Autodesk Inventor part; units mm, degrees
ref_plane "YZ Plane" through (0, 0, 0) normal (1, 0, 0) x (0, 1, 0)
ref_plane "XZ Plane" through (0, 0, 0) normal (0, 1, 0) x (-1, 0, 0)
ref_plane "XY Plane" through (0, 0, 0) normal (0, 0, 1) x (1, 0, 0)
sketch "Sketch1" plane through (0, 0, 0) normal (0, 1, 0) x (-1, 0, 0)
  circle A0 centre (0, 0) radius 1.25
  line L0 (0, 0) -> (-58, 0) construction
  line L1 (0, 0) -> (58, 0) construction
  circle A1 centre (-58, 0) radius 1.25
  line L2 (0, 0) -> (0, -23) construction
  line L3 (0, 0) -> (23, 0) construction
  line L4 (0, -23) -> (-58, -23) construction
  line L5 (-58, -23) -> (-58, 0) construction
  circle A2 centre (-58, -23) radius 1.25
  circle A3 centre (0, -23) radius 1.25
  line L6 (-61.5, 3.5) -> (3.5, 3.5)
  line L7 (3.5, 3.5) -> (3.5, -26.5)
  line L8 (3.5, -26.5) -> (-61.5, -26.5)
  line L9 (-61.5, -26.5) -> (-61.5, 3.5)
  line L10 (-61.5, 3.5) -> (3.5, -26.5) construction
  line L11 (3.5, 3.5) -> (-61.5, -26.5) construction
  circle A4 centre (0, 0) radius 2
  circle A5 centre (0, -23) radius 2
  circle A6 centre (-58, -23) radius 2
  circle A7 centre (-58, 0) radius 2
  line L12 (3.5, 3.5) -> (-61.5, 3.5)
  line L13 (-61.5, 3.5) -> (-61.5, 4)
  line L14 (-61.5, 4) -> (3.5, 4)
  line L15 (3.5, 4) -> (3.5, 3.5)
  line L16 (3.5, 4) -> (-28.25, 4)
  line L17 (-28.25, 4) -> (-28.25, 23.05)
  line L18 (-28.25, 23.05) -> (3.5, 23.05)
  line L19 (3.5, 23.05) -> (3.5, 4)
  line L20 (-58, -11.5) -> (0, -11.5) construction
  line L21 (-29, -23) -> (-29, 0) construction
  line L22 (3.5, 23.05) -> (-1.58, 23.05)
  line L23 (-1.58, 23.05) -> (-1.58, 20.51) construction
  line L24 (-1.58, 20.51) -> (3.5, 20.51) construction
  line L25 (3.5, 20.51) -> (3.5, 23.05)
  circle A8 centre (-1.58, 20.51) radius 1.016
  line L26 (3.5, 4) -> (-1.58, 4)
  line L27 (-1.58, 4) -> (-1.58, 6.54) construction
  line L28 (-1.58, 6.54) -> (3.5, 6.54) construction
  line L29 (3.5, 6.54) -> (3.5, 4)
  line L30 (-28.25, 4) -> (-25.71, 4)
  line L31 (-25.71, 4) -> (-25.71, 6.54) construction
  line L32 (-25.71, 6.54) -> (-28.25, 6.54) construction
  line L33 (-28.25, 6.54) -> (-28.25, 4)
  line L34 (-28.25, 23.05) -> (-25.71, 23.05)
  line L35 (-25.71, 23.05) -> (-25.71, 20.51) construction
  line L36 (-25.71, 20.51) -> (-28.25, 20.51) construction
  line L37 (-28.25, 20.51) -> (-28.25, 23.05)
  circle A9 centre (-25.71, 20.51) radius 1.016
  circle A10 centre (-25.71, 6.54) radius 1.016
  circle A11 centre (-1.58, 6.54) radius 1.016
  circle A12 centre (-1.58, 20.51) radius 1.905
  circle A13 centre (-1.58, 6.54) radius 1.905
  circle A14 centre (-25.71, 6.54) radius 1.905
  circle A15 centre (-25.71, 20.51) radius 1.905
  line L38 (3.5, -26.5) -> (-61.5, -26.5)
  line L39 (-61.5, -26.5) -> (-61.5, -27)
  line L40 (-61.5, -27) -> (3.5, -27)
  line L41 (3.5, -27) -> (3.5, -26.5)
  line L42 (3.5, -27) -> (-58.65, -27)
  line L43 (-58.65, -27) -> (-58.65, -65)
  line L44 (-58.65, -65) -> (3.5, -65)
  line L45 (3.5, -65) -> (3.5, -27)
  line L46 (3.5, 23.05) -> (4, 23.05)
  line L47 (4, 23.05) -> (4, -65)
  line L48 (4, -65) -> (3.5, -65)
  line L49 (3.5, -65) -> (3.5, 23.05)
  line L50 (4, -65) -> (36, -65)
  line L51 (36, -65) -> (36, 22)
  line L52 (36, 22) -> (4, 22)
  line L53 (4, 22) -> (4, -65)
  line L54 (36, -21.5) -> (4, -21.5) construction
  line L55 (20, -65) -> (20, 22) construction
  line L56 (7.5, -61.5) -> (32.5, -61.5) construction
  line L57 (32.5, -61.5) -> (32.5, 18.5) construction
  line L58 (32.5, 18.5) -> (7.5, 18.5) construction
  line L59 (7.5, 18.5) -> (7.5, -61.5) construction
  line L60 (7.5, -61.5) -> (32.5, 18.5) construction
  line L61 (32.5, -61.5) -> (7.5, 18.5) construction
  circle A16 centre (32.5, 18.5) radius 1.5
  circle A17 centre (7.5, 18.5) radius 1.5
  circle A18 centre (7.5, -61.5) radius 1.5
  circle A19 centre (32.5, -61.5) radius 1.5
  circle A20 centre (32.5, 18.5) radius 2.5
  circle A21 centre (7.5, 18.5) radius 2.5
  circle A22 centre (32.5, -61.5) radius 2.5
  circle A23 centre (7.5, -61.5) radius 2.5
  line L62 (4, 23.05) -> (-28.25, 23.05)
  line L63 (-28.25, 23.05) -> (-28.25, 23.55)
  line L64 (-28.25, 23.55) -> (4, 23.55)
  line L65 (4, 23.55) -> (4, 23.05)
  line L66 (36, 22) -> (36.5, 22)
  line L67 (36.5, 22) -> (36.5, -65)
  line L68 (36.5, -65) -> (36, -65)
  line L69 (36, -65) -> (36, 22)
  line L70 (36.5, -65) -> (-58.65, -65)
  line L71 (-58.65, -65) -> (-58.65, -65.5)
  line L72 (-58.65, -65.5) -> (36.5, -65.5)
  line L73 (36.5, -65.5) -> (36.5, -65)
  line L74 (-61.5, 4) -> (-62, 4)
  line L75 (-62, 4) -> (-62, -27)
  line L76 (-62, -27) -> (-61.5, -27)
  line L77 (-61.5, -27) -> (-61.5, 4)
  line L78 (-62, 23.55) -> (36.5, 23.55)
  line L79 (36.5, 23.55) -> (36.5, -65.5)
  line L80 (36.5, -65.5) -> (-62, -65.5)
  line L81 (-62, -65.5) -> (-62, 23.55)
  line L82 (-65, 26.55) -> (39.5, 26.55)
  line L83 (39.5, 26.55) -> (39.5, -68.5)
  line L84 (39.5, -68.5) -> (-65, -68.5)
  line L85 (-65, -68.5) -> (-65, 26.55)
  line L86 (3.5, 3.5) -> (-8, 3.5)
  line L87 (-8, 3.5) -> (-8, -26.5) construction
  line L88 (-8, -26.5) -> (3.5, -26.5)
  line L89 (3.5, -26.5) -> (3.5, 3.5)
  line L90 (-11.75, -7.75) -> (-4.25, -7.75)
  line L91 (-4.25, -7.75) -> (-4.25, -15.25)
  line L92 (-4.25, -15.25) -> (-11.75, -15.25)
  line L93 (-11.75, -15.25) -> (-11.75, -7.75)
  line L94 (-11.75, -7.75) -> (-4.25, -15.25) construction
  line L95 (-4.25, -7.75) -> (-11.75, -15.25) construction
  point P0 (-29, -11.5)
  point P1 (20, -21.5)
  point P2 (-8, -11.5)
  dimension "d0" = 2.5
  dimension "d1" = 58
  dimension "d2" = 180
  dimension "d3" = 2.5
  dimension "d4" = 23
  dimension "d5" = 270
  dimension "d6" = 90
  dimension "d7" = 2.5
  dimension "d8" = 2.5
  dimension "d9" = 65
  dimension "d10" = 30
  dimension "d11" = 4
  dimension "d12" = 4
  dimension "d13" = 4
  dimension "d14" = 4
  dimension "d15" = 0.5
  dimension "d16" = 31.75
  dimension "d17" = 19.05
  dimension "d18" = 5.08
  dimension "d19" = 2.54
  dimension "d20" = 2.032
  dimension "d21" = 5.08
  dimension "d22" = 2.54
  dimension "d23" = 2.54
  dimension "d24" = 2.54
  dimension "d25" = 2.54
  dimension "d26" = 2.54
  dimension "d27" = 2.032
  dimension "d28" = 2.032
  dimension "d29" = 2.032
  dimension "d30" = 3.81
  dimension "d31" = 3.81
  dimension "d32" = 3.81
  dimension "d33" = 3.81
  dimension "d34" = 0.5
  dimension "d35" = 62.15
  dimension "d36" = 38
  dimension "d37" = 0.5
  dimension "d38" = 32
  dimension "d39" = 87
  dimension "d40" = 25
  dimension "d41" = 80
  dimension "d42" = 3
  dimension "d43" = 3
  dimension "d44" = 3
  dimension "d45" = 3
  dimension "d46" = 5
  dimension "d47" = 5
  dimension "d48" = 5
  dimension "d49" = 5
  dimension "d50" = 0.5
  dimension "d51" = 0.5
  dimension "d52" = 0.5
  dimension "d53" = 0.5
  dimension "d56" = 3
  dimension "d59" = 11.5
  dimension "d60" = 7.5
  dimension "d61" = 7.5
extrude "Extrusion1" add sketch "Sketch1" against normal blind 2 contours A0 | A1 | A2 | A3 | L13 L14 L15 L6 | L6 L7 L8 L9 | L9 L39 L76 L75 L74 L13 | L8 L41 L40 L39 | L74 L81 L78 L63 L17 L14 | L15 L19 L46 L47 L48 L45 L41 L7 | L40 L43 L71 L80 L81 L76 | L17 L18 L19 L14 | L40 L45 L44 L43 | L44 L48 L50 L68 L73 L72 L71 | L64 L65 L46 L18 L63 | L78 L79 L66 L52 L47 L65 | L47 L52 L51 L50 | L51 L66 L67 L68 | A4 | A5 | A6 | A7 | A8 | A9 | A10 | A11 | A12 | A13 | A14 | A15 | A16 | A17 | A18 | A19 | A20 | A21 | A22 | A23 | L82 L83 L84 L85 | L90 L91 L92 L93
extrude "Extrusion2" add sketch "Sketch1" along normal blind 15 contours L82 L83 L84 L85
extrude "Extrusion3" cut sketch "Sketch1" against normal up to surface (2 mm away) contours L90 L91 L92 L93
extrude "Extrusion4" add sketch "Sketch1" along normal blind 5.5 contours A20 | A21 | A22 | A23
extrude "Extrusion5" add sketch "Sketch1" along normal blind 8.5 contours A16 | A17 | A18 | A19
extrude "Extrusion6" add sketch "Sketch1" along normal blind 3 contours A4 | A5 | A6 | A7
extrude "Extrusion7" add sketch "Sketch1" along normal blind 6 contours A0 | A1 | A2 | A3
extrude "Extrusion8" add sketch "Sketch1" along normal blind 2.5 contours A12 | A13 | A14 | A15
extrude "Extrusion9" add sketch "Sketch1" along normal blind 5 contours A8 | A9 | A10 | A11
sketch "Sketch2" plane through (65, -2, 26.55) normal (1, 0, 0) x (0, 0, -1)
  line L0 (28.55, 5) -> (24.55, 5)
  line L1 (51.55, 5) -> (47.55, 5)
  line L2 (24.55, 5) -> (51.55, 5) construction
  line L3 (44.05, 8) -> (32.05, 8)
  line L4 (32.05, 8) -> (32.05, 2)
  line L5 (32.05, 2) -> (44.05, 2)
  line L6 (44.05, 2) -> (44.05, 8)
  line L7 (44.05, 8) -> (32.05, 2) construction
  line L8 (32.05, 8) -> (44.05, 2) construction
  line L9 (44.05, 8) -> (56.05, 8) construction
  point P0 (26.55, 2)
  point P1 (38.05, 5)
  dimension "d76" = 12
  dimension "d77" = 180
extrude "Extrusion10" cut sketch "Sketch2" against normal up to surface (3 mm away)
sketch "Sketch3" plane through (0, 15, 0) normal (0, 1, 0) x (1, 0, 0)
  circle A0 centre (25.71, -6.54) radius 1.905
  circle A1 centre (1.58, -6.54) radius 1.905
  circle A2 centre (25.71, -20.51) radius 1.905
  circle A3 centre (1.58, -20.51) radius 1.905
  circle A4 centre (58, 23) radius 2
  circle A5 centre (0, 23) radius 2
  circle A6 centre (58, 0) radius 2
  circle A7 centre (0, 0) radius 2
  circle A8 centre (-32.5, 61.5) radius 2.5
  circle A9 centre (-32.5, -18.5) radius 2.5
  circle A10 centre (-7.5, 61.5) radius 2.5
  circle A11 centre (-7.5, -18.5) radius 2.5
  line L0 (11.75, 15.25) -> (11.75, 7.75)
  line L1 (11.75, 7.75) -> (4.25, 7.75)
  line L2 (4.25, 7.75) -> (4.25, 15.25)
  line L3 (4.25, 15.25) -> (11.75, 15.25)
  line L4 (62, 65.5) -> (-36.5, 65.5)
  line L5 (-36.5, 65.5) -> (-36.5, -23.55)
  line L6 (-36.5, -23.55) -> (62, -23.55)
  line L7 (62, -23.55) -> (62, 5.5)
  line L8 (65, 5.5) -> (62, 5.5)
  line L9 (65, 17.5) -> (65, 5.5)
  line L10 (65, 17.5) -> (62, 17.5)
  line L11 (62, 17.5) -> (62, 65.5)
  line L12 (62, 5.5) -> (64, 5.5)
  line L13 (64, 5.5) -> (64, 17.5)
  line L14 (64, 17.5) -> (62, 17.5)
  line L15 (62, 17.5) -> (62, 5.5)
  dimension "d80" = 2
extrude "Extrusion11" cut sketch "Sketch3" against normal up to surface (9 mm away) contours L10 L13 L8 L15
fillet "Fillet1" radius 3.175 4 edges at (65, 6.5, 26.55) (65, 6.5, -68.5) (-39.5, 6.5, -68.5) (-39.5, 6.5, 26.55)
properties part number "Enclosure"
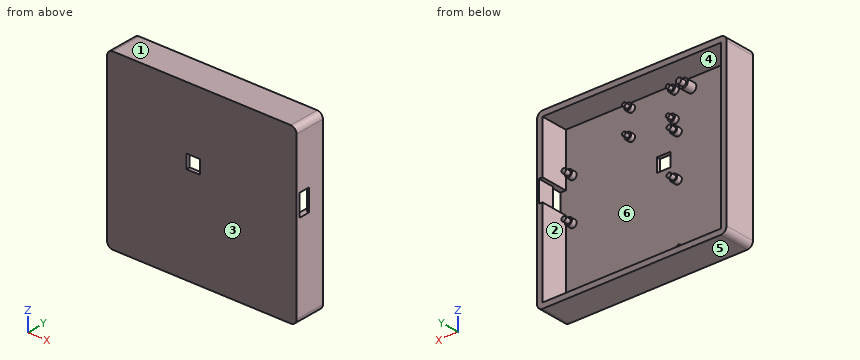
Work out the finished part from the listing and answer in its coordinate system (mm). Face numbers are marked on the shaded views. A direction names the side the tool comes from. Coordinates: 2 decimals unless noted, no trailing zeros. Order: outer loops, then holes, each group sorted by start corner. A loop starts at its lowest first (then second) coordinate and runs counter-clockwise, first axis right, second up. Notation, with made-up numbers: (48, 59.25) - (56, 59.25) arc R23 ccw to (56, 77.25) - close; hole circle Ø10 at (-20, 14). An arc over 180 degrees is marked (long way). Answer as a JSON object with one key per item and string values.
1. Each of these flat-tipped pins is pushed along its axis until it touches: P1, Ø5, axis at x = -4, z = -9, coming from the +Y side; P2, Ø1.2, axis at x = 0, z = -0.5, coming from the +Y side; P3, Ø3, axis at x = 2.5, z = 6.5, coming from the +Y side. Where does it stop, or does it pass through?
Output values:
{"P1": "stops at y = 0", "P2": "stops at y = 6", "P3": "stops at y = 5"}
2. Consider line 1 (Z direction, x = 11.5, y = 7.25); line 2 (X direction, y = 2.5, z = -63.5); line 3 (X direction, y = 11.5, z = -34). Determine where each line is inside the solid, lowest interval first.
Output values:
{"line 1": "z = -68.5 to -65.5, 23.55 to 26.55", "line 2": "x = -39.5 to -36.5, -34 to -31, -9 to -6, 62 to 65", "line 3": "x = -39.5 to -36.5, 62 to 65"}
3. A tool of negligible diameter and unlimited length cuts with its end or side. For the marked faces 1 and 2, from which of +Z, -Z, +X, -X, +Y, -Y can it reach the whole face along a straight path? Write none if from no direction.
Output values:
{"face 1": "+Z, +X, -X, +Y, -Y", "face 2": "+Y"}
4. Find section B-B on y = 10.25. Determine the outline of the cut face in (x, z) (3 decimals), plus the area to 3 significant figures.
Output values:
{"outline": "(-39.5, -65.325) arc R3.175 ccw to (-36.325, -68.5) - (61.825, -68.5) arc R3.175 ccw to (65, -65.325) - (65, 23.375) arc R3.175 ccw to (61.825, 26.55) - (-36.325, 26.55) arc R3.175 ccw to (-39.5, 23.375) - close; hole (-36.5, -65.5) - (62, -65.5) - (62, -17.5) - (64, -17.5) - (64, -5.5) - (62, -5.5) - (62, 23.55) - (-36.5, 23.55) - close", "area": "1,130 mm²"}
5. Find section C-C on x = -32.5. Determine the outline of the cut face in (y, z).
Output values:
{"outline": "(-2, -68.5) - (15, -68.5) - (15, -65.5) - (0, -65.5) - (0, -64) - (5.5, -64) - (5.5, -63) - (8.5, -63) - (8.5, -60) - (5.5, -60) - (5.5, -59) - (0, -59) - (0, 16) - (5.5, 16) - (5.5, 17) - (8.5, 17) - (8.5, 20) - (5.5, 20) - (5.5, 21) - (0, 21) - (0, 23.55) - (15, 23.55) - (15, 26.55) - (-2, 26.55) - close"}
6. The mould has two halves that part along Z. Classify the marked faces 3, 4, 5 and 6: +Z half, -Z half, draft (parallel to the pull), parting line (faces both ways), or undercut.
Output values:
{"face 3": "draft", "face 4": "undercut", "face 5": "-Z half", "face 6": "undercut"}
7. Find section A-A on z = -10.5. Determine the outline of the cut face in (x, y).
Output values:
{"outline": "(-39.5, -2) - (4.25, -2) - (4.25, 0) - (-36.5, 0) - (-36.5, 15) - (-39.5, 15) - close; (11.75, -2) - (65, -2) - (65, 0) - (11.75, 0) - close; (64, 6) - (65, 6) - (65, 15) - (64, 15) - close"}
8. Find section D-D on z = -23. Determine the outline of the cut face in (x, y).
Output values:
{"outline": "(-39.5, -2) - (65, -2) - (65, 15) - (62, 15) - (62, 0) - (60, 0) - (60, 3) - (59.25, 3) - (59.25, 6) - (56.75, 6) - (56.75, 3) - (56, 3) - (56, 0) - (2, 0) - (2, 3) - (1.25, 3) - (1.25, 6) - (-1.25, 6) - (-1.25, 3) - (-2, 3) - (-2, 0) - (-36.5, 0) - (-36.5, 15) - (-39.5, 15) - close"}
